For this review, take the finished solid that the model builds, in its own axes (mm). A direction names the side the tool comes from. Coordinates: 2 decimals unless noted, no trailing zeros. Loops run counter-clockwise (first coordinate to the right, second up) from the corner with the lowest first, then second, coordinate; pieces in that order, holes last. Notation, with made-up numbers: (-18.5, 79) - (4.5, 79) arc R24 ccw to (4.5, 115) - close; hole circle Ø9 at (77.5, -29). An arc over 180 degrees is marked (long way). One line per item, written item: value. Start each with the question number.
1. The part is to be moulded in two halves that separate along Y. For faces 4 (the face through (-68, -16, 5)), 5 (the face through (18, 0, 5)), 6 (the face through (-56, 25, 5)), say which applies: released by +Y, released by -Y, zero draft, split by the parting line, or undercut.
2. Take a section at C-C, the plane x = -50. State the section outline as (y, z) points, and give its area (3 significant figures).
3. To check wall thickness, follow line 1 (Y direction, x = -50, z = 7); line 2 (Y direction, x = 0, z = 4.5); line 3 (Y direction, x = -88.5, z = 34). State the ranges of each line that lie inside material, in increasing order. Write a range as from..to.
4. For faces 1 (the face through (-68, 17, 5)), 2 (the face through (-20.16, -22.83, 4.93)), 3 (the face through (-31, -1, 0)), list the 3-axis set-ups (+Z, -Z, +X, -X, +Y, -Y) from which the entire face can be reached by the end or side of a thin tool; tool diameter is ignored.
5. Take a section at B-B, the plane z = 20. State the section outline as (x, y) points, and give its area (3 significant figures).
6. Take a section at D-D, the plane y = -26.5. State the section outline as (x, z) points, and give its area (3 significant figures).
7. Insertion check: pin 1 (19 mm diameter, centred on x = -50, y = 25, fed in from +Z); pin 2 (2 mm diameter, centred on x = -97, z = 5, fed in from +Y); pin 3 (12 mm diameter, centred on y = -3.5, z = 4.5, fed in from -X). Each pin has a flat end and moves straight along its axis. Give the tip position at first contact, or say it passes through.
8. Take a section at A-A, the plane y = 0. State the section outline as (x, z) points, and give its area (3 significant figures).
```python
from build123d import *

# Parameters (mm, degrees)
F0_R          = 6
F1_DEPTH      = 10
F2_R          = 10
F3_DEPTH      = 8
F3_DEPTH_BACK = 8
F4_R          = 6
F5_DEPTH      = 25


with BuildPart() as f1:
    # F0 (on Top) → F1 (new body)
    with BuildSketch(Plane.XY):
        with BuildLine():
            ThreePointArc((-35.6, -35.8), (-19.901005, -22.69799), (0, -18))
            ThreePointArc((0, -18), (18, 0), (0, 18))
            ThreePointArc((0, 18), (-20.182572, 22.254358), (-36.930589, 34.293449))
            ThreePointArc((-36.930589, 34.293449), (-55.383923, 39.40414), (-68, 25))
            Line((-68, 25), (-68, -25))
            ThreePointArc((-68, -25), (-55.6921, -42.076299), (-35.6, -35.8))
        make_face()
        with Locations((-50, -25)):
            Circle(F0_R, mode=Mode.SUBTRACT)
        with Locations((-50, 25)):
            Circle(F0_R, mode=Mode.SUBTRACT)
        Circle(F0_R, mode=Mode.SUBTRACT)
    extrude(amount=F1_DEPTH)

    # F2 (on Front) → F3 (join, two sides)
    with BuildSketch(Plane.XZ) as f3_sk:
        with BuildLine():
            Line((-105.07352, 0), (-6, 0))
            Line((-6, 0), (-6, 9.523888))
            ThreePointArc((-6, 9.523888), (-15.894485, 9.37036), (-25.770109, 10))
            ThreePointArc((-25.770109, 10), (-61.725464, 19.270605), (-93.371199, 38.69428))
            ThreePointArc((-93.371199, 38.69428), (-127.749328, 30.547983), (-110, 0))
            Line((-110, 0), (-105.07352, 0))
        make_face()
        with Locations((-107.53676, 21.861666)):
            Circle(F2_R, mode=Mode.SUBTRACT)
        with BuildLine():
            ThreePointArc((-25.770109, 10), (-15.894485, 9.37036), (-6, 9.523888))
            Line((-6, 9.523888), (-6, 10))
            Line((-6, 10), (-25.770109, 10))
        make_face()
        with BuildLine():
            Line((-6, 10), (-6, 9.523888))
            ThreePointArc((-6, 9.523888), (-2.997134, 9.725826), (0, 10))
            Line((0, 10), (-6, 10))
        make_face()
        with BuildLine():
            ThreePointArc((-110, 0), (-107.53676, -0.138334), (-105.07352, 0))
            Line((-105.07352, 0), (-110, 0))
        make_face()
    extrude(amount=F3_DEPTH)
    extrude(f3_sk.sketch, amount=-F3_DEPTH_BACK)

    # F4 (on face) → F5 (cut)
    with BuildSketch(Plane(origin=(0, 0, 0), x_dir=(1, 0, 0), z_dir=(0, 0, -1))):
        Circle(F4_R)
    extrude(amount=-F5_DEPTH, mode=Mode.SUBTRACT)


solid = f1.part
```
Solutions:
1. face 4: zero draft
1. face 5: split by the parting line
1. face 6: undercut
2. outline: (-43, 0) - (-31, 0) - (-31, 10) - (-43, 10) - close; (-19, 0) - (19, 0) - (19, 10) - (8, 10) - (8, 14.97) - (-8, 14.97) - (-8, 10) - (-19, 10) - close; (31, 0) - (40.16, 0) - (40.16, 10) - (31, 10) - close
2. area: 671 mm2
3. line 1: -43..-31, -19..19, 31..40.16
3. line 2: -18..-6, 6..18
3. line 3: -8..8
4. face 1: +Z, -Z, -X, +Y
4. face 2: +Z, -Z, +X, -Y
4. face 3: -Z, +X, +Y, -Y
5. outline: (-129.46, -8) - (-117.36, -8) - (-117.36, 8) - (-129.46, 8) - close; (-97.71, -8) - (-63.41, -8) - (-63.41, 8) - (-97.71, 8) - close
5. area: 742 mm2
6. outline: (-67.94, 0) - (-55.81, 0) - (-55.81, 10) - (-67.94, 10) - close; (-44.19, 0) - (-26.16, 0) - (-26.16, 10) - (-44.19, 10) - close
6. area: 302 mm2
7. pin 1: z = 10
7. pin 2: y = 8
7. pin 3: x = -126.38
8. outline: (-110, 0) arc R22 ccw to (-105.07, 0) - (-6, 0) - (-6, 10) - (-25.77, 10) arc R125 cw to (-93.37, 38.69) arc R22 ccw (long way) to start; (6, 0) - (18, 0) - (18, 10) - (6, 10) - close; hole circle Ø20 at (-107.54, 21.86)
8. area: 2,740 mm2
